Part print with two shaded views. Sizes in mm from the minimum x, y, z corner. A direction names the side the tool comes from. Round coordinates to 2 decimals unless told otherwise and drop trailing zeros. Loops run counter-clockwise (first coordinate to the right, second up) from the corner with the lowest first, then second, coordinate; pieces in that order, holes last. Notation, with made-up numbers: M 79,-17.75 L 90,-17.75 A29 cw 90,11.25 Z; hole C 9.25,21.5 d5. An arc over 180 degrees is marked long. Answer as CSV lines item,"result". Start each with the question number.
Item 1: Which spindle directions (+Z, -Z, +X, -X, +Y, -Y) get a long thin tool onto all of the face, cutting with end or side? Do the marked faces 1, 2, 3 and 4. Say none if no direction does.
Item 2: Band-saw the part on A-A (y = 97). Give the cut face in (x, z), and give its area (3 significant figures).
Item 3: Drop flat-ended pins along their axis: pin 1 Ø3 at (y, z) = (19.5, 9) entering from -X; pin 2 Ø10 at (x, y) = (23, 17) entering from -Z; pin 3 Ø1.8 at (x, z) = (39, 7.5) entering from +Y; pin 4 Ø1.8 at (x, y) = (39, 22) entering from +Z. Give the stop position or say it passes through.
Item 4: Wall check: line 1 (Y direction, x = 24, z = 10); line 2 (Y direction, x = 37, z = 5.5); line 3 (X direction, y = 43, z = 9.5). Give the ranges that are in metal, low to high.
Item 5: Band-saw the part on B-B (x = 32.5). Give the cut face in (y, z), and give its area (3 significant figures).
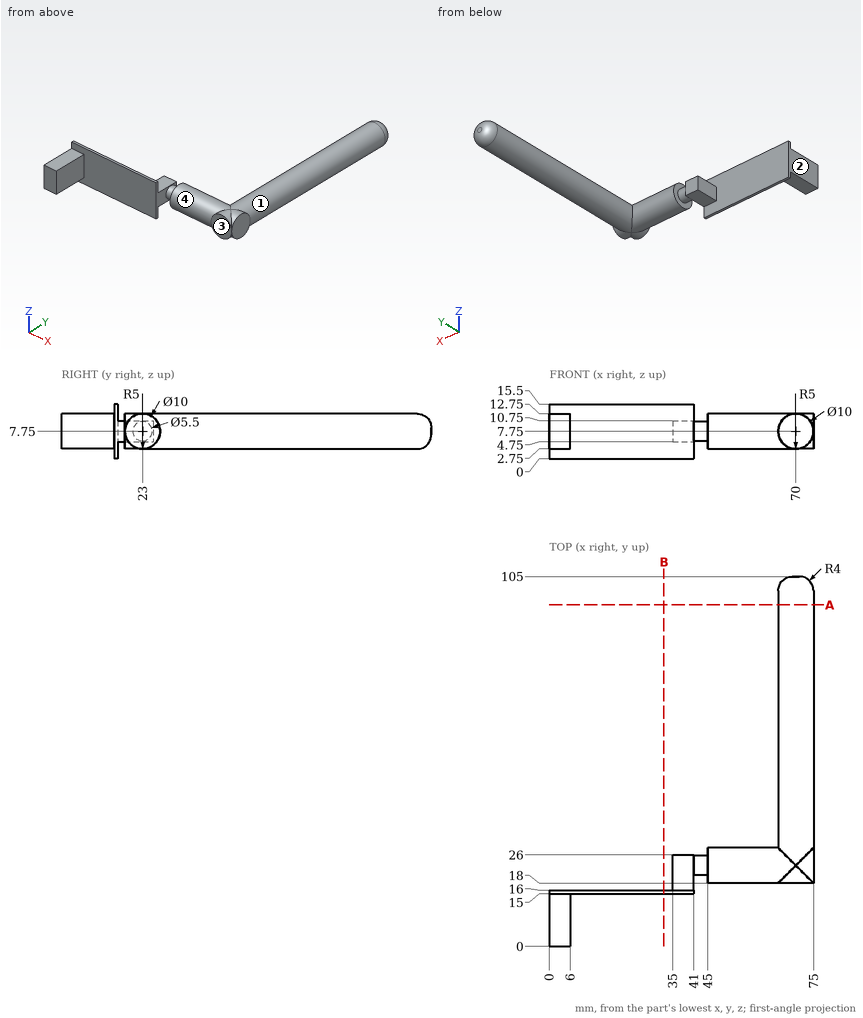
Answer block:
1,face 1,"+Y"
1,face 2,"+Z, -Z, -X, +Y, -Y"
1,face 3,"+Z, -Z, +X, -Y"
1,face 4,"none"
2,outline,"C 70,7.75 d10"
2,area,"78.5 mm^2"
3,pin 1,"stops at x = 35"
3,pin 2,"stops at z = 0"
3,pin 3,"stops at y = 26"
3,pin 4,"stops at z = 10.75"
4,line 1,"y = 15 to 16"
4,line 2,"y = 15 to 26"
4,line 3,"x = 65.32 to 74.68"
5,outline,"M 15,0 L 16,0 L 16,15.5 L 15,15.5 Z"
5,area,"15.5 mm^2"
